from build123d import *

# Parameters (mm, degrees)
BOSS_EXTRU_1_DEPTH                            = 47
ESQUISSE2_W                                   = 17
ESQUISSE2_H                                   = 14.999999999999986
ENL_V_MAT_EXTRU_1_DEPTH                       = 87.8691544795966
BOSS_EXTRU_2_DEPTH                            = 27.72
BOSS_EXTRU_2_DEPTH_BACK                       = 18.78
BOSS_EXTRU_5_REACH                            = 154.075
BOSS_EXTRU_5_DIRECTION_2_REACH                = 154.075
ESQUISSE5_R                                   = 1.2499999999999978
ENL_V_MAT_EXTRU_2_DEPTH                       = 121.28542019885793
ESQUISSE6_W                                   = 15.000000000000004
ESQUISSE6_H                                   = 11.999999999999996
ENL_V_MAT_EXTRU_3_DEPTH                       = 10
CONG_1_R                                      = 2
CONG_2_R                                      = 3
ESQUISSE9_R                                   = 3.4290000000000016
ENL_V_MAT_EXTRU_4_DEPTH                       = 123.34009215468092
TROU_POUR_TARAUDAGE_POUR_TROU_TARAUD_M5_REACH = 160.94
TROU_POUR_TARAUDAGE_POUR_TROU_TARAUD_2_R      = 2.1
CONG_3_R                                      = 2


with BuildPart() as part:
    # Esquisse1 → Boss.-Extru.1 (new body)
    with BuildSketch(Plane.XY):
        with BuildLine():
            Line((-15, 63.999998751364224), (0, 63.999998751364224))
            Line((0, 63.999998751364224), (-4.3e-16, -63.999998751364224))
            ThreePointArc((-4.3e-16, -63.999998751364224), (-7.499998751364213, -71.5), (-14.999999999999986, -64.00000124863578))
            Line((-14.999999999999986, -64.00000124863578), (-15, 63.999998751364224))
        make_face()
    extrude(amount=BOSS_EXTRU_1_DEPTH)

    # Esquisse2 → Enlèv. mat.-Extru.1 (cut, through all)
    with BuildSketch(Plane.ZY.offset(14.999999999999993)):
        with Locations((23.5, -64.00000000000009)):
            Rectangle(ESQUISSE2_W, ESQUISSE2_H)
        Polygon((47, 63.999998751364224), (31, 63.999998751364224), (31, -41.50000000000009), (47.000000000000014, -41.50000000000009), align=None)
        Polygon((0, 63.999998751364224), (16, 63.999998751364224), (16, -41.5000000000001), (1.292e-14, -41.5000000000001), align=None)
    extrude(amount=-ENL_V_MAT_EXTRU_1_DEPTH, mode=Mode.SUBTRACT)

    # Esquisse3 → Boss.-Extru.2 (add, two sides: drawn at the far end of the back side and taken through both)
    with BuildSketch(Plane.ZY.offset(14.999999999999993).offset(-BOSS_EXTRU_2_DEPTH_BACK)):
        Polygon((38.358000000000004, 103.28494444213939), (38.35800000000001, 66.67694444213939), (8.642, 66.67694444213939), (8.642, 103.28494444213939), (5.641999999999999, 103.28494444213939), (5.642000000000004, 63.676944442139366), (41.35800000000001, 63.676944442139366), (41.358000000000004, 103.28494444213939), align=None)
    extrude(amount=BOSS_EXTRU_2_DEPTH + BOSS_EXTRU_2_DEPTH_BACK)

    # Boss.-Extru.5: up to this face of the body (flat: up to its plane)
    boss_extru_5_end = Plane(part.part.faces().sort_by_distance((-19.47, 103.284944442, 7.142))[0])
    # Esquisse4 → Boss.-Extru.5 (add, up to the picked face)
    with BuildSketch(Plane(origin=(-7.29e-15, 66.67694444213939, 0), x_dir=(1, 1.1e-16, 0), z_dir=(-1.1e-16, 1, 0)), mode=Mode.PRIVATE) as boss_extru_5_sk1:
        Polygon((3.780000000000016, -5.641999999999999), (6.780000000000015, -5.641999999999999), (6.780000000000019, -41.358000000000004), (3.780000000000016, -41.358000000000004), align=None)
    boss_extru_5_tool1 = split(extrude(boss_extru_5_sk1.sketch, amount=BOSS_EXTRU_5_REACH, mode=Mode.PRIVATE), bisect_by=boss_extru_5_end, keep=Keep.BOTH, mode=Mode.PRIVATE)
    # Esquisse4 → Boss.-Extru.5 (add, up to the picked face)
    with BuildSketch(Plane(origin=(-7.29e-15, 66.67694444213939, 0), x_dir=(1, 1.1e-16, 0), z_dir=(-1.1e-16, 1, 0)), mode=Mode.PRIVATE) as boss_extru_5_sk2:
        Polygon((-42.719999999999985, -5.641999999999999), (-45.71999999999999, -5.641999999999999), (-45.719999999999985, -41.358000000000004), (-42.719999999999985, -41.358000000000004), align=None)
    boss_extru_5_tool2 = split(extrude(boss_extru_5_sk2.sketch, amount=BOSS_EXTRU_5_REACH, mode=Mode.PRIVATE), bisect_by=boss_extru_5_end, keep=Keep.BOTH, mode=Mode.PRIVATE)
    add(boss_extru_5_tool1.solids().sort_by(Axis((5.28, 66.676944, 23.5), (-1.1e-16, 1, 0)))[0])
    add(boss_extru_5_tool2.solids().sort_by(Axis((-44.22, 66.676944, 23.5), (-1.1e-16, 1, 0)))[0])

    # Boss.-Extru.5 direction 2: up to this face of the body (flat: up to its plane)
    boss_extru_5_direction_2_end = Plane(part.part.faces().sort_by_distance((-21.345791374, 63.676944442, 23.5))[0])
    # Esquisse4 → Boss.-Extru.5 direction 2 (add, up to the picked face)
    with BuildSketch(Plane(origin=(-7.29e-15, 66.67694444213939, 0), x_dir=(1, 1.1e-16, 0), z_dir=(-1.1e-16, 1, 0)), mode=Mode.PRIVATE) as boss_extru_5_direction_2_sk1:
        Polygon((3.780000000000016, -5.641999999999999), (6.780000000000015, -5.641999999999999), (6.780000000000019, -41.358000000000004), (3.780000000000016, -41.358000000000004), align=None)
    boss_extru_5_direction_2_tool1 = split(extrude(boss_extru_5_direction_2_sk1.sketch, amount=-BOSS_EXTRU_5_DIRECTION_2_REACH, mode=Mode.PRIVATE), bisect_by=boss_extru_5_direction_2_end, keep=Keep.BOTH, mode=Mode.PRIVATE)
    # Esquisse4 → Boss.-Extru.5 direction 2 (add, up to the picked face)
    with BuildSketch(Plane(origin=(-7.29e-15, 66.67694444213939, 0), x_dir=(1, 1.1e-16, 0), z_dir=(-1.1e-16, 1, 0)), mode=Mode.PRIVATE) as boss_extru_5_direction_2_sk2:
        Polygon((-42.719999999999985, -5.641999999999999), (-45.71999999999999, -5.641999999999999), (-45.719999999999985, -41.358000000000004), (-42.719999999999985, -41.358000000000004), align=None)
    boss_extru_5_direction_2_tool2 = split(extrude(boss_extru_5_direction_2_sk2.sketch, amount=-BOSS_EXTRU_5_DIRECTION_2_REACH, mode=Mode.PRIVATE), bisect_by=boss_extru_5_direction_2_end, keep=Keep.BOTH, mode=Mode.PRIVATE)
    add(boss_extru_5_direction_2_tool1.solids().sort_by(Axis((5.28, 66.676944, 23.5), (1.1e-16, -1, 0)))[0])
    add(boss_extru_5_direction_2_tool2.solids().sort_by(Axis((-44.22, 66.676944, 23.5), (1.1e-16, -1, 0)))[0])

    # Esquisse5 → Enlèv. mat.-Extru.2 (cut, through all)
    with BuildSketch(Plane.XY.offset(41.358000000000025)):
        with Locations(Location((-11.469999999999994, 92.28494444213936, 0), (0, 0, 270))):
            Circle(ESQUISSE5_R)
        with Locations(Location((-35.47, 92.28494444213936, 0), (0, 0, 270))):
            Circle(ESQUISSE5_R)
    extrude(amount=-ENL_V_MAT_EXTRU_2_DEPTH, mode=Mode.SUBTRACT)

    # Esquisse6 → Enlèv. mat.-Extru.3 (cut)
    with BuildSketch(Plane.XZ.offset(-63.676944442139366)):
        Polygon((-17.335036050217354, 41.35800000000002), (-2.335036050217353, 41.35800000000002), (-2.3350360502173517, 29.35800000000002), (-17.335036050217354, 29.35800000000002), align=None)
        with Locations((-9.835036050217353, 11.642000000000012)):
            Rectangle(ESQUISSE6_W, ESQUISSE6_H)
    extrude(amount=-ENL_V_MAT_EXTRU_3_DEPTH, mode=Mode.SUBTRACT)

    # Congé1
    cong_1_edges = [part.edges().sort_by_distance(p)[0] for p in [
        (-15, 63.67694444213936, 23.500000000000014),
        (-1.167518025108679, 63.676944442139366, 31),
        (0, 63.676944442139366, 23.5),
        (-1.167518025108679, 63.676944442139366, 16),
    ]]
    fillet(cong_1_edges, radius=CONG_1_R)

    # Congé2
    cong_2_edges = [part.edges().sort_by_distance(p)[0] for p in [
        (-7.499999999999994, -41.50000000000009, 31),
        (-7.499999999999994, -41.5000000000001, 16),
    ]]
    fillet(cong_2_edges, radius=CONG_2_R)

    # Esquisse9 → Enlèv. mat.-Extru.4 (cut, through all)
    with BuildSketch(Plane.XY.offset(47)):
        with Locations((-7.499999999999992, -64)):
            Circle(ESQUISSE9_R)
    extrude(amount=-ENL_V_MAT_EXTRU_4_DEPTH, mode=Mode.SUBTRACT)

    # Trou pour taraudage pour trou taraud 2 → Trou pour taraudage pour trou taraudé M52 (cut, up to next)
    with BuildSketch(Plane(origin=(4.53e-15, -41.5000000000001, 0), x_dir=(1, 1.1e-16, 0), z_dir=(-1.1e-16, 1, 0)), mode=Mode.PRIVATE) as trou_pour_taraudage_pour_trou_taraud_m5_sk1:
        with Locations((-7.5, -8.642)):
            Circle(TROU_POUR_TARAUDAGE_POUR_TROU_TARAUD_2_R)
    trou_pour_taraudage_pour_trou_taraud_m5_tool1 = extrude(trou_pour_taraudage_pour_trou_taraud_m5_sk1.sketch, amount=-TROU_POUR_TARAUDAGE_POUR_TROU_TARAUD_M5_REACH, mode=Mode.PRIVATE) & part.part
    # Trou pour taraudage pour trou taraud 2 → Trou pour taraudage pour trou taraudé M52 (cut, up to next)
    with BuildSketch(Plane(origin=(4.53e-15, -41.5000000000001, 0), x_dir=(1, 1.1e-16, 0), z_dir=(-1.1e-16, 1, 0)), mode=Mode.PRIVATE) as trou_pour_taraudage_pour_trou_taraud_m5_sk2:
        with Locations((-7.5, -38.358)):
            Circle(TROU_POUR_TARAUDAGE_POUR_TROU_TARAUD_2_R)
    trou_pour_taraudage_pour_trou_taraud_m5_tool2 = extrude(trou_pour_taraudage_pour_trou_taraud_m5_sk2.sketch, amount=-TROU_POUR_TARAUDAGE_POUR_TROU_TARAUD_M5_REACH, mode=Mode.PRIVATE) & part.part
    add(trou_pour_taraudage_pour_trou_taraud_m5_tool1.solids().sort_by_distance((-7.5, -41.5, 8.642))[0], mode=Mode.SUBTRACT)
    add(trou_pour_taraudage_pour_trou_taraud_m5_tool2.solids().sort_by_distance((-7.5, -41.5, 38.358))[0], mode=Mode.SUBTRACT)

    # Congé3
    # the kernel refuses this fillet: 2 mm, written as the material it takes off along each edge
    with BuildSketch(Plane(origin=(-19.919245368957963, 63.676944442139366, 16), x_dir=(1.1e-16, -1, 0), z_dir=(1, 1.1e-16, 0))) as cong_3_piece_1:
        with BuildLine():
            CenterArc((1.9676981475831852, -2), CONG_3_R, 90, 79.68848194075031)
            Line((5.6133e-13, -1.6420000000001131), (0, 0))
            Line((0, 0), (1.9676981475831852, 0))
        make_face()
    extrude(amount=17.584209318740605, mode=Mode.SUBTRACT)
    with BuildSketch(Plane(origin=(-15, 63.67694444213936, 17.64200000000001), x_dir=(0, -1, 0), z_dir=(0, 0, -1))) as cong_3_piece_2:
        with BuildLine():
            CenterArc((CONG_3_R, -CONG_3_R), CONG_3_R, 90, 90)
            Line((0, -CONG_3_R), (0, 0))
            Line((0, 0), (CONG_3_R, 0))
        make_face()
    extrude(amount=6.64200000000001, mode=Mode.SUBTRACT)
    with BuildSketch(Plane(origin=(-19.919245368957963, 63.676944442139366, 31), x_dir=(1.1e-16, -1, 0), z_dir=(1, 1.1e-16, 0))) as cong_3_piece_3:
        with BuildLine():
            CenterArc((1.967698147583178, 2), CONG_3_R, 190.31151805925052, 79.68848194074951)
            Line((5.6133e-13, 1.6420000000000847), (0, 0))
            Line((0, 0), (1.967698147583178, 0))
        make_face()
    extrude(amount=17.584209318740605, mode=Mode.SUBTRACT)
    with BuildSketch(Plane(origin=(-15, 63.67694444213936, 36.00000000000001), x_dir=(0, -1, 0), z_dir=(0, 0, -1))) as cong_3_piece_4:
        with BuildLine():
            CenterArc((CONG_3_R, -CONG_3_R), CONG_3_R, 90, 90)
            Line((0, -CONG_3_R), (0, 0))
            Line((0, 0), (CONG_3_R, 0))
        make_face()
    extrude(amount=6.641999999999989, mode=Mode.SUBTRACT)


solid = part.part
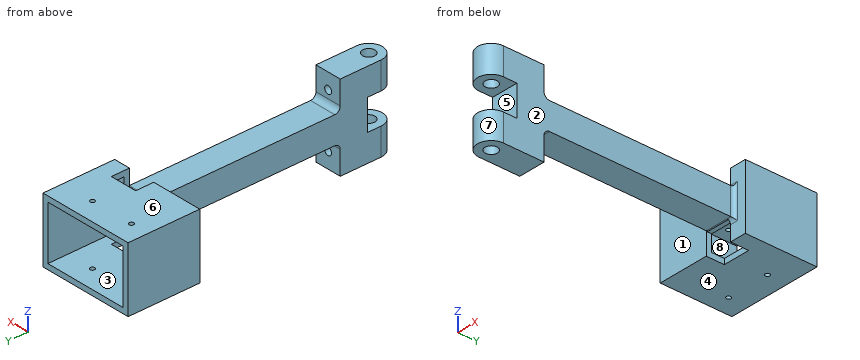
Design review of the part built by this model. Coordinates are the model's own, in mm. Face numbers are marked on the shaded views. A direction names the side the tool comes from. Round coordinates to 2 decimals unless told otherwise and drop trailing zeros. Write each loop counter-clockwise with the first axis right and the second up, starting at its lowest first coordinate (ties: lowest second). Pieces come first, ordered by that corner, then holes. Notation, with made-up numbers: (55, 71.5) - (97, 71.5) arc R13 cw to (97, 86.5) - close; hole circle Ø10 at (57, -4.5). An arc over 180 degrees is marked (long way). Return JSON: item names as keys, results as strings. Group by question number.
Item 1: The part is to be moulded in two halves that separate along X. For the marked faces 6, 7 and 8, say which applies: pulls with the +X half, pulls with the -X half, needs draft (parallel to the pull), parting line crosses it, or undercut.
Item 2: We need section D-D on y = 15. Write out the cut boundary in (x, z).
Item 3: Insertion check: P1, Ø10, axis at x = 2.5, z = 29, coming from the -Y side; P2, Ø1, axis at x = -13, z = 33.5, coming from the -Y side; P3, Ø1.5, axis at y = -17, z = 26, coming from the -X side. Each pin has a flat end and moves straight along its axis. Give the tip position at first contact, or say it passes through.
Item 4: We need section C-C on x = -7.5. Give the number of separate pieces and of enclosed holes in the cut face, and give its area (3 significant figures).
Item 5: We need section A-A on z = 24. Write out the cut boundary in (x, y), and give its area (3 significant figures).
Item 6: For probe 1 along Z at (x, y) = (-41, 74); probe 2 along Y at (x, z) = (-7, 42.5); probe 3 along X at (y, z) = (89, 13.5), list the stretches that pass through material, from the lowest coordinate up. Write a range as [from, to].
Item 7: We need section B-B on x = -31.5. Write out the cut boundary in (y, z).
Item 8: Machinability: for the marked faces 1, 2, 3, 4 and 5, which of the approach directions +Z, -Z, +X, -X, +Y, -Y give a long, thin tool a straight path to every point of the face, cutting with its end or side? Answer none if there is none.
Model answer:
{
 "1": {"face 6": "needs draft", "face 7": "parting line crosses it", "face 8": "undercut"},
 "2": {"outline": "(-15, 16) - (0, 16) - (0, 31) - (-15, 31) - close"},
 "3": {"P1": "stops at y = -68.5", "P2": "stops at y = -69.59", "P3": "stops at x = -15"},
 "4": {"separate pieces": "7", "enclosed holes": "0", "area": "2,580 mm²"},
 "5": {"outline": "(-45.72, 63.68) - (-17, 63.68) arc R2 cw to (-15, 61.68) - (-15, -56.5) - (0, -56.5) - (0, 61.68) arc R2 cw to (2, 63.68) - (6.78, 63.68) - (6.78, 103.28) - (3.78, 103.28) - (3.78, 66.68) - (-42.72, 66.68) - (-42.72, 103.28) - (-45.72, 103.28) - close", "area": "2,180 mm²"},
 "6": {"probe 1": "z = [5.64, 8.64], [38.36, 41.36]", "probe 2": "y = [-71.48, -67.39], [-60.61, -41.5]", "probe 3": "x = [-45.72, -42.72], [3.78, 6.78]"},
 "7": {"outline": "(63.68, 5.64) - (103.28, 5.64) - (103.28, 8.64) - (66.68, 8.64) - (66.68, 38.36) - (103.28, 38.36) - (103.28, 41.36) - (63.68, 41.36) - close"},
 "8": {"face 1": "+Z, -Z, -X, -Y", "face 2": "+Z, -Z, +X, -Y", "face 3": "+Y", "face 4": "-Z, +X, -X, +Y", "face 5": "+X, -X, -Y"}
}
